Job drawing, mm, ordinate dimensions from the low corner. One solid piece. Round coordinates to 2 decimals unless told otherwise and drop trailing zeros. Order: outer loops, then holes, each group sorted by start corner. A loop starts at its lowest first (then second) coordinate and runs counter-clockwise, first axis right, second up. Notation, with made-up numbers: (-20.75, 69.25) -> (16.25, 69.25) arc R12 ccw to (16.25, 90.25) -> close; hole circle Ø10 at (1.5, 87). An arc over 180 degrees is marked (long way). Return JSON: item names as keys, results as strings. Group by question number.
Q1. Cut at A-A (y = 45.5). Write the cut outline in (x, z).
Q2. Flat gauge pin, fed straight in: pin 1 (3 mm diameter, centred on x = 22, y = 45.5, fed in from +Z). Where does the tip first touch, or does it go through?
Q3. Probe line 1 along Y through (x, z) = (22, 5.25); line 2 along Y through (x, z) = (37.5, 8.25); line 3 along X through (y, z) = (15, 3.5). List the from-to ranges inside material, lowest first.
Q4. Cut at B-B (x = 37.5). Write the cut outline in (y, z), then the cut area to 3 significant figures.
Q5. Cut at C-C (y = 30). Write the cut outline in (x, z).
Q6. Cut at D-D (z = 3). Write the cut outline in (x, y), then the cut area to 3 significant figures.
Q7. Mould opens along Y. For the marked faces 1, 2, 3 and 4 say: +Y half, -Y half, draft (parallel to the pull), parting line (faces both ways), or undercut.
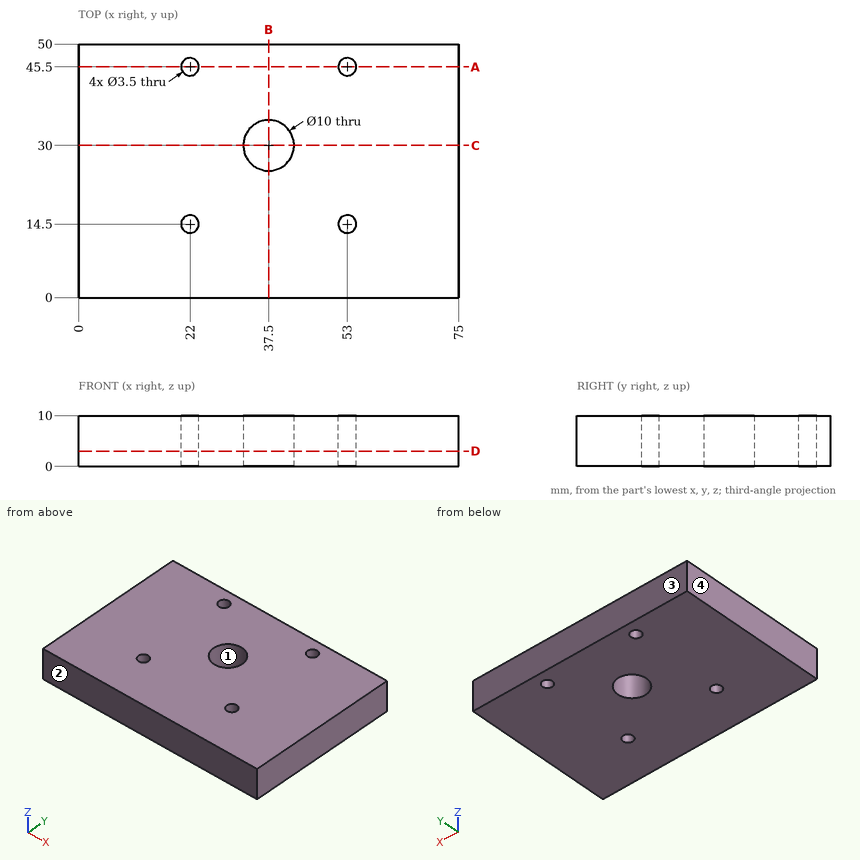
Solution:
{
 "1": {"outline": "(0, 0) -> (20.25, 0) -> (20.25, 10) -> (0, 10) -> close; (23.75, 0) -> (51.25, 0) -> (51.25, 10) -> (23.75, 10) -> close; (54.75, 0) -> (75, 0) -> (75, 10) -> (54.75, 10) -> close"},
 "2": {"pin 1": "passes through"},
 "3": {"line 1": "y = 0 to 12.75, 16.25 to 43.75, 47.25 to 50", "line 2": "y = 0 to 25, 35 to 50", "line 3": "x = 0 to 20.32, 23.68 to 51.32, 54.68 to 75"},
 "4": {"outline": "(0, 0) -> (25, 0) -> (25, 10) -> (0, 10) -> close; (35, 0) -> (50, 0) -> (50, 10) -> (35, 10) -> close", "area": "400 mm²"},
 "5": {"outline": "(0, 0) -> (32.5, 0) -> (32.5, 10) -> (0, 10) -> close; (42.5, 0) -> (75, 0) -> (75, 10) -> (42.5, 10) -> close"},
 "6": {"outline": "(0, 0) -> (75, 0) -> (75, 50) -> (0, 50) -> close; hole circle Ø3.5 at (22, 14.5); hole circle Ø3.5 at (22, 45.5); hole circle Ø10 at (37.5, 30); hole circle Ø3.5 at (53, 14.5); hole circle Ø3.5 at (53, 45.5)", "area": "3,630 mm²"},
 "7": {"face 1": "undercut", "face 2": "-Y half", "face 3": "+Y half", "face 4": "draft"}
}
